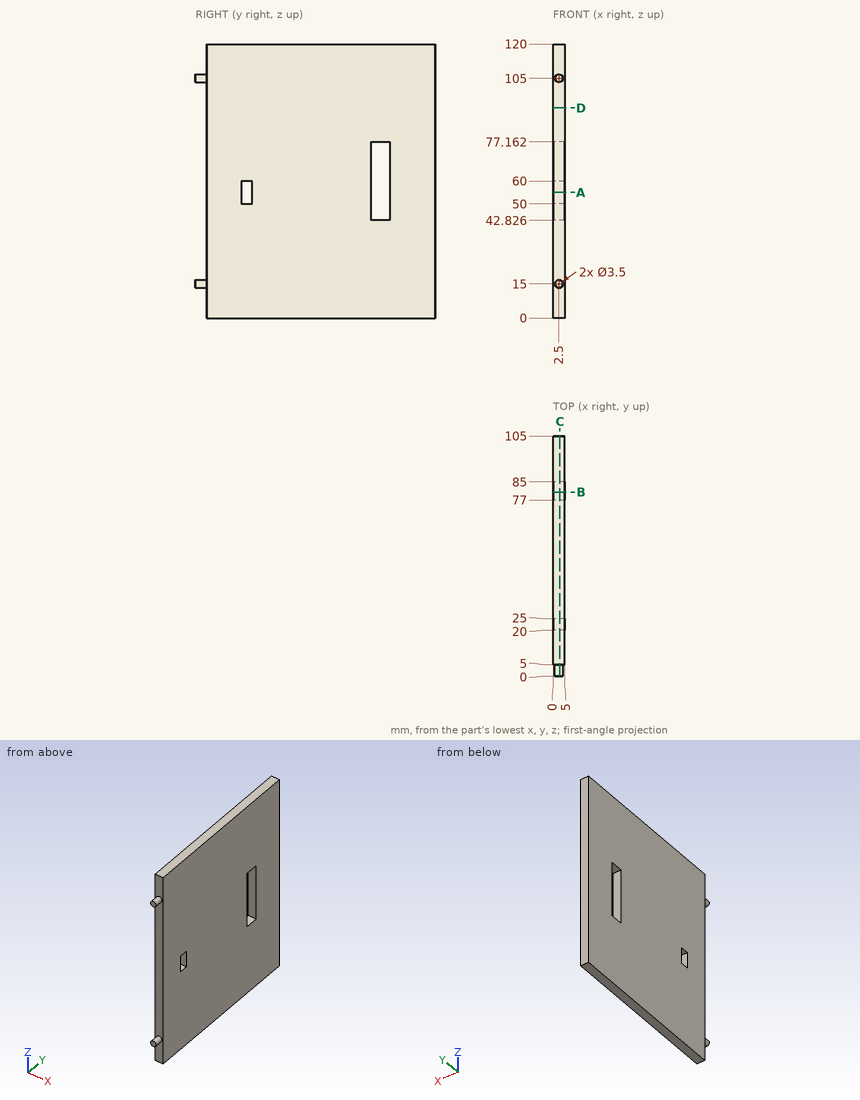
Here's the drawing with two shaded views (mm, measured from the low corner). I have some questions. Give positions to 0.01 mm unless a question says otherwise; leave off trailing zeros. Loops run counter-clockwise (first coordinate to the right, second up) from the corner with the lowest first, then second, coordinate; pieces in that order, holes last. Notation, with made-up numbers: (51, 77) - (72, 77) arc R18 ccw to (72, 108) - close; hole circle Ø10 at (-39.75, -18). An arc over 180 degrees is marked (long way). Answer in a Markdown table with one row per item. Add a question column.
Q1. If we section it at A-A (z = 55): List the corners of the cut face in (x, y) for me, plus the area to 3 significant figures.
Q2. If we section it at D-D (z = 92): List the corners of the cut face in (x, y) for me.
Q3. If we section it at C-C (x = 2.95): List the corners of the cut face in (y, z) for me, plus the area to 3 significant figures.
Q4. If we section it at B-B (y = 80.5): List the corners of the cut face in (x, z) for me.
Q5. Please list where these lines run through material, in increasing order: L1, parallel to Y at x = 1.8, z = 76; L2, parallel to Y at x = 2.2, z = 9.5; L3, parallel to Z at x = 4.6, y = 79.5. Write a range as from..to.
Q6. For pin 1 (1 mm diameter, centred on x = 4, y = 20.5, fed in from -Z); pin 2 (3 mm diameter, centred on x = 2, z = 93.5, fed in from -Y), each with a flat end and sliding along its axis, tell me the tip position at first contact or that it passes through.
The answers:
| question | item | result |
|---|---|---|
| 1 | outline | (0, 5) - (5, 5) - (5, 20) - (0, 20) - close; (0, 25) - (5, 25) - (5, 77) - (0, 77) - close; (0, 85) - (5, 85) - (5, 105) - (0, 105) - close |
| 1 | area | 435 mm^2 |
| 2 | outline | (0, 5) - (5, 5) - (5, 105) - (0, 105) - close |
| 3 | outline | (0, 13.31) - (5, 13.31) - (5, 0) - (105, 0) - (105, 120) - (5, 120) - (5, 106.69) - (0, 106.69) - (0, 103.31) - (5, 103.31) - (5, 16.69) - (0, 16.69) - close; hole (20, 50) - (25, 50) - (25, 60) - (20, 60) - close; hole (77, 42.83) - (85, 42.83) - (85, 77.16) - (77, 77.16) - close |
| 3 | area | 11,700 mm^2 |
| 4 | outline | (0, 0) - (5, 0) - (5, 42.83) - (0, 42.83) - close; (0, 77.16) - (5, 77.16) - (5, 120) - (0, 120) - close |
| 5 | L1 | y = 5..77, 85..105 |
| 5 | L2 | y = 5..105 |
| 5 | L3 | z = 0..42.83, 77.16..120 |
| 6 | pin 1 | stops at z = 0 |
| 6 | pin 2 | stops at y = 5 |
